For this review, take the finished solid that the model builds, in its own axes (mm). A direction names the side the tool comes from. Coordinates: 2 decimals unless noted, no trailing zeros. Write each loop counter-clockwise with the first axis right and the second up, starting at its lowest first coordinate (ties: lowest second). Pieces come first, ordered by that corner, then holes. Notation, with made-up numbers: (70, 86) - (111, 86) arc R14 ccw to (111, 100) - close; hole circle Ø3 at (39, 58). An arc over 180 degrees is marked (long way). Use one line per item in the form item = value. Start each with the question number.
1) Mouldability with a two-part tool opening along X and no side actions: class faces 1 (the flat face through (7.7, -8, -39)), 2 (the flat face through (-5, -58, -39)), 3 (the flat face through (-2.7, -56, -40)) as pulls with the +X half, pulls with the -X half, needs draft (parallel to the pull), parting line crosses it, or undercut.
2) We need section C-C (z = 13). Give the boundary of the cut face in (x, y), plus the area to 3 significant figures.
3) We need section B-B (y = -12). Give the boundary of the cut face in (x, z).
4) We need section D-D (z = -10.5). Give the boundary of the cut face in (x, y).
5) Tool access review of faces 4 (the flat face through (2.7, -8, -40)), 5 (the flat face through (-0.1, -70, -36.3)), 6 (the flat face through (6, -9, -42.1)), 7 (the flat face through (-7.7, -56, -39)), 8 (the flat face through (-1, 108, -1)): name each direction out of +Z, -Z, +X, -X, +Y, -Y from which nothing blocks a thin tool from reaching the whole face with its end or side.
6) For L1, parallel to X at y = -7.5, z = -36.5; L2, parallel to Y at x = 5.2, z = -39.25; L3, parallel to X at y = 66.5, z = 0.5, list the stretches that pass through material, from the lowest coordinate up. Write a range as from..to.
7) We need section A-A (x = 0). Give the boundary of the cut face in (y, z), plus the area to 3 significant figures.
8) Insertion check: P1, Ø6, axis at x = -18.5, z = -3, coming from the -Y side; P2, Ø3, axis at y = 65, z = -33, coming from the +X side; P3, Ø1.4, axis at x = 5.2, y = -7.5, coming from the -Z side; P4, Ø2.5, axis at y = -8.5, z = -40, coming from the -X side. Each pin has a flat end and moves straight along its axis. Give the tip position at first contact, or say it passes through.
```python
from build123d import *

# Parameters (mm, degrees)
SKETCH_1_R               = 37
EXTRUDE_1_DEPTH          = 110
EXTRUDE_1_DEPTH_BACK     = 70
SKETCH_2_R               = 36
CUT_EXTRUDE_1_DEPTH      = 108
CUT_EXTRUDE_1_DEPTH_BACK = 70
CUT_EXTRUDE_6_DEPTH      = 70
SKETCH_7_W               = 22
SKETCH_7_H               = 20
CUT_EXTRUDE_7_DEPTH      = 43
SKETCH_10_W              = 8
SKETCH_10_H              = 12
CUT_EXTRUDE_8_DEPTH      = 8.1
SKETCH_12_W              = 5
SKETCH_12_H              = 5
SKETCH_12_R              = 1.15
EXTRUDE_3_DEPTH          = 1
EXTRUDE_3_DEPTH_BACK     = 5.1
SKETCH_13_R              = 1.15
CUT_EXTRUDE_9_DEPTH      = 18.4


with BuildPart() as part:
    # 草圖1 → 填料-伸長1 (new body, two sides)
    with BuildSketch(Plane(origin=(0, 0, 0), x_dir=(1, 0, 0), z_dir=(0, 1, 0))) as extrude_1_sk:
        Circle(SKETCH_1_R)
    extrude(amount=EXTRUDE_1_DEPTH)
    extrude(extrude_1_sk.sketch, amount=-EXTRUDE_1_DEPTH_BACK)

    # 草圖2 → 除料-伸長1 (cut, two sides)
    with BuildSketch(Plane(origin=(0, 0, 0), x_dir=(1, 0, 0), z_dir=(0, 1, 0))) as cut_extrude_1_sk:
        Circle(SKETCH_2_R)
    extrude(amount=CUT_EXTRUDE_1_DEPTH, mode=Mode.SUBTRACT)
    extrude(cut_extrude_1_sk.sketch, amount=-CUT_EXTRUDE_1_DEPTH_BACK, mode=Mode.SUBTRACT)

    # 草圖6 → 除料-伸長6 (cut)
    with BuildSketch(Plane(origin=(0, 0, 0), x_dir=(1, 0, 0), z_dir=(0, 1, 0))):
        with BuildLine():
            Line((-36, 0), (26.300758937, 0))
            Line((26.300758937, 0), (36, 0))
            ThreePointArc((36, 0), (33.645512806, 12.805446811), (26.890029553, 23.935879149))
            Line((26.890029553, 23.935879149), (27.509698295, 24.743009108))
            ThreePointArc((27.509698295, 24.743009108), (34.546047798, 13.25030496), (37, 0))
            ThreePointArc((37, 0), (0, -37), (-37, 0))
            ThreePointArc((-37, 0), (-34.546047798, 13.25030496), (-27.509698295, 24.743009108))
            Line((-27.509698295, 24.743009108), (-26.890029553, 23.935879149))
            ThreePointArc((-26.890029553, 23.935879149), (-33.645512806, 12.805446811), (-36, 0))
        make_face()
    extrude(amount=-CUT_EXTRUDE_6_DEPTH, mode=Mode.SUBTRACT)

    # 草圖7 → 除料-伸長7 (cut)
    with BuildSketch(Plane(origin=(0, -10, 0), x_dir=(1, 0, 0), z_dir=(0, 1, 0))):
        with Locations((0, 27.910624132)):
            Rectangle(SKETCH_7_W, SKETCH_7_H)
    extrude(amount=-CUT_EXTRUDE_7_DEPTH, mode=Mode.SUBTRACT)

    # 草圖10 → 除料-伸長8 (cut)
    with BuildSketch(Plane(origin=(0, 110, 0), x_dir=(1, 0, 0), z_dir=(0, 1, 0))):
        with Locations((-13.992241726, -15.397733401)):
            Rectangle(SKETCH_10_W, SKETCH_10_H)
        with Locations((13.992241726, -15.397733401)):
            Rectangle(SKETCH_10_W, SKETCH_10_H)
    extrude(amount=-CUT_EXTRUDE_8_DEPTH, mode=Mode.SUBTRACT)

    # 草圖12 → 填料-伸長3 (add, two sides)
    with BuildSketch(Plane.XY.offset(-37)) as extrude_3_sk:
        with Locations((-5.2, -7.5)):
            Rectangle(SKETCH_12_W, SKETCH_12_H)
        with Locations((-5.2, -7.5)):
            Circle(SKETCH_12_R, mode=Mode.SUBTRACT)
        with Locations((5.2, -7.5)):
            Rectangle(SKETCH_12_W, SKETCH_12_H)
        with Locations((5.2, -7.5)):
            Circle(SKETCH_12_R, mode=Mode.SUBTRACT)
        with Locations((5.2, -55.5)):
            Rectangle(SKETCH_12_W, SKETCH_12_H)
        with Locations((5.2, -55.5)):
            Circle(SKETCH_12_R, mode=Mode.SUBTRACT)
        with Locations((-5.2, -55.5)):
            Rectangle(SKETCH_12_W, SKETCH_12_H)
        with Locations((-5.2, -55.5)):
            Circle(SKETCH_12_R, mode=Mode.SUBTRACT)
    extrude(amount=EXTRUDE_3_DEPTH)
    extrude(extrude_3_sk.sketch, amount=-EXTRUDE_3_DEPTH_BACK)

    # 草圖13 → 除料-伸長9 (cut)
    with BuildSketch(Plane.XY.offset(-37)):
        with Locations((5.2, -7.5)):
            Circle(SKETCH_13_R)
        with Locations((-5.2, -7.5)):
            Circle(SKETCH_13_R)
        with Locations((-5.2, -55.5)):
            Circle(SKETCH_13_R)
        with Locations((5.2, -55.5)):
            Circle(SKETCH_13_R)
    extrude(amount=CUT_EXTRUDE_9_DEPTH, mode=Mode.SUBTRACT)


solid = part.part
```
Determined:
q1.face_1 = pulls with the +X half
q1.face_2 = needs draft
q1.face_3 = undercut
q2.outline = (-34.64, 0) - (-33.57, 0) - (-33.57, 108) - (-17.99, 108) - (-17.99, 110) - (-34.64, 110) - close; (-9.99, 108) - (9.99, 108) - (9.99, 110) - (-9.99, 110) - close; (17.99, 108) - (33.57, 108) - (33.57, 0) - (34.64, 0) - (34.64, 110) - (17.99, 110) - close
q2.area = 338 mm²
q3.outline = (-27.51, -24.74) arc R37 ccw to (-11, -35.33) - (-11, -34.28) arc R36 cw to (-26.89, -23.94) - close; (11, -35.33) arc R37 ccw to (27.51, -24.74) - (26.89, -23.94) arc R36 cw to (11, -34.28) - close
q4.outline = (-35.48, 0) - (-34.43, 0) - (-34.43, 108) - (34.43, 108) - (34.43, 0) - (35.48, 0) - (35.48, 110) - (-35.48, 110) - close
q5.face_4 = -Z, +Y, -Y
q5.face_5 = +Z, -Z, +X, -X, -Y
q5.face_6 = -Z, +X, -X, +Y, -Y
q5.face_7 = -Z, -X, +Y, -Y
q5.face_8 = -Y
q6.L1 = -7.7..-6.35, -4.05..4.05, 6.35..7.7
q6.L2 = -58..-56.65, -54.35..-53, -10..-8.65, -6.35..-5
q6.L3 = -37..-36, 36..37
q7.outline = (-70, -37) - (-53, -37) - (-53, -36) - (-70, -36) - close; (-10, -37) - (110, -37) - (110, 37) - (0, 37) - (0, 36) - (108, 36) - (108, -36) - (-10, -36) - close
q7.area = 391 mm²
q8.P1 = 108
q8.P2 = 19.41
q8.P3 = through
q8.P4 = -7.7
